Source: CAD feature listing. Evaluate the final solid. Frame: model axes, mm. A direction names the side the tool comes from. Round coordinates to 2 decimals unless told otherwise and drop trailing zeros. Order: outer loops, then holes, each group sorted by start corner. A loop starts at its lowest first (then second) coordinate and runs counter-clockwise, first axis right, second up. Notation, with made-up numbers: M 11.5,45.25 L 62.5,45.25 A27 ccw 62.5,65.25 Z; hole C -19.75,63 d10. An arc over 180 degrees is marked long. Answer as CSV lines item,"result". Start each with the question number.
Item 1: Section query A-A on z = 0. Return the cut outline in (x, y), plus the area to 3 significant figures.
Item 2: Section query C-C on x = 9.5. Return the cut outline in (y, z), plus the area to 3 significant figures.
Item 3: Set-up query: faces 4 (the face through (1, 0, 3)), 5 (the face through (-57, 0, 0)), 6 (the face through (12, 1.429, 0)). Return all of +Z, -Z, +X, -X, +Y, -Y with unobstructed straight access to the full face (end or side cutting, diameter ignored); none if empty.
Item 4: Line query: line 1 (X direction, y = -9, z = -7.25); line 2 (X direction, y = 0.5, z = -8.25); line 3 (Y direction, x = -2.25, z = -8.5). Output: solid intervals per line, ascending. Write a range as [from, to].
Item 5: Pull-direction query (Y, two-part tool) for faces 1 (the face through (-28.1, -11, -5.72)), 2 (the face through (0, -3, -3)), 3 (the face through (-2.46, -0.49, -9.67)); classes: +Y half, -Y half, draft (parallel to the pull), parting line (faces both ways), or undercut.
Item 6: First-contact query: P1, Ø0.8, axis at x = 12, z = 0.5, coming from the +Y side; P2, Ø1.5, axis at y = 0, z = 8.5, coming from the +X side; P3, Ø5, axis at y = 1.5, z = -7.5, coming from the +X side. Flat tips, straight axial feed; report the tip coordinate or a pass-through.
Item 7: Section query D-D on x = -44. Return the cut outline in (y, z).
Item 8: Section query B-B on y = 0. Return the cut outline in (x, z).
from build123d import *

# Parameters (mm, degrees)
SKETCH1_R           = 12.4
BOSS_EXTRUDE1_DEPTH = 57
SKETCH2_R           = 3
BOSS_EXTRUDE2_DEPTH = 2.3
SKETCH3_R           = 2
BOSS_EXTRUDE3_DEPTH = 15.5
SKETCH4_R           = 1.27
CUT_EXTRUDE1_DEPTH  = 5
CUT_EXTRUDE3_DEPTH  = 12.7


with BuildPart() as part:
    # Sketch1 → Boss-Extrude1 (new body)
    with BuildSketch(Plane(origin=(0, 0, 0), x_dir=(0, 0, -1), z_dir=(1, 0, 0))):
        Circle(SKETCH1_R)
    extrude(amount=-BOSS_EXTRUDE1_DEPTH)

    # Sketch2 → Boss-Extrude2 (add)
    with BuildSketch(Plane(origin=(0, 0, 0), x_dir=(0, 0, -1), z_dir=(1, 0, 0))):
        Circle(SKETCH2_R)
    extrude(amount=BOSS_EXTRUDE2_DEPTH)

    # Sketch3 → Boss-Extrude3 (add)
    with BuildSketch(Plane(origin=(2.3, 0, 0), x_dir=(0, 0, -1), z_dir=(1, 0, 0))):
        Circle(SKETCH3_R)
    extrude(amount=BOSS_EXTRUDE3_DEPTH)

    # Sketch4 → Cut-Extrude1 (cut)
    with BuildSketch(Plane(origin=(0, 0, 0), x_dir=(0, 0, -1), z_dir=(1, 0, 0))):
        with Locations((8.5, 0)):
            Circle(SKETCH4_R)
        with Locations((-8.5, 0)):
            Circle(SKETCH4_R)
    extrude(amount=-CUT_EXTRUDE1_DEPTH, mode=Mode.SUBTRACT)

    # Sketch5 → Cut-Extrude3 (cut)
    with BuildSketch(Plane(origin=(17.8, 0, 0), x_dir=(0, 0, -1), z_dir=(1, 0, 0))):
        with BuildLine():
            Line((0, 1.429), (-1.399270882, 1.429))
            ThreePointArc((-1.399270882, 1.429), (0, 2), (1.399270882, 1.429))
            Line((1.399270882, 1.429), (0, 1.429))
        make_face()
    extrude(amount=-CUT_EXTRUDE3_DEPTH, mode=Mode.SUBTRACT)


solid = part.part
Results:
1,outline,"M -57,-12.4 L 0,-12.4 L 0,-3 L 2.3,-3 L 2.3,-2 L 17.8,-2 L 17.8,1.43 L 5.1,1.43 L 5.1,2 L 2.3,2 L 2.3,3 L 0,3 L 0,12.4 L -57,12.4 Z"
1,area,"1,480 mm^2"
2,outline,"M 1.43,-1.4 L 1.43,1.4 A2 ccw long Z"
2,area,"11.5 mm^2"
3,face 4,"+X"
3,face 5,"+Z, -Z, -X, +Y, -Y"
3,face 6,"+Z, -Z, +X, +Y"
4,line 1,"[-57, 0]"
4,line 2,"[-57, -5]"
4,line 3,"[-9.03, -1.27], [1.27, 9.03]"
5,face 1,"parting line"
5,face 2,"draft"
5,face 3,"undercut"
6,P1,"y = 1.43"
6,P2,"x = -5"
6,P3,"x = 0"
7,outline,"C 0,0 d24.8"
8,outline,"M -57,-12.4 L 0,-12.4 L 0,-9.77 L -5,-9.77 L -5,-7.23 L 0,-7.23 L 0,-3 L 2.3,-3 L 2.3,-2 L 17.8,-2 L 17.8,2 L 2.3,2 L 2.3,3 L 0,3 L 0,7.23 L -5,7.23 L -5,9.77 L 0,9.77 L 0,12.4 L -57,12.4 Z"
